CAD build for the part. Positions are in the model's coordinates, mm. Face numbers are marked on the shaded views. A direction names the side the tool comes from. Coordinates: 2 decimals unless noted, no trailing zeros. Write each loop counter-clockwise with the first axis right and the second up, starting at its lowest first coordinate (ties: lowest second). Pieces come first, ordered by that corner, then holes. Notation, with made-up numbers: (56.25, 20) - (65.25, 20) arc R7 ccw to (65.25, 26) - close; hole circle Ø4 at (-30.5, 80.25). An arc over 180 degrees is marked (long way). One line per question, with ' | ' between items. Start each with the question number.
1. Which spindle directions (+Z, -Z, +X, -X, +Y, -Y) get a long thin tool onto all of the face, cutting with end or side? Do the marked faces 1, 2 and 3. Say none if no direction does.
2. Probe line 1 (Z direction, x = -3.5, y = 4); line 2 (X direction, y = -22, z = -5); line 3 (X direction, y = -14, z = -11.5). List the from-to ranges inside material, lowest first.
3. Band-saw the part on A-A, the plane z = -6.35. Give the number of separate pieces and of enclosed holes in the cut face, then the cut area to 3 significant figures.
4. Flat gauge pins, fed straight in: P1, Ø6, axis at x = -19.5, z = -5, coming from the +Y side; P2, Ø4, axis at x = -22, y = -3.5, coming from the +Z side; P3, Ø0.8, axis at x = -31, z = -6.5, coming from the +Y side; P4, Ø1.4, axis at y = 5.5, z = -11, coming from the +X side. Where does each tip first touch, or does it go through?
5. Two-plate mould, pull along Z, no slides. Class the marked faces 4, 5, 6 and 7: +Z half, -Z half, draft (parallel to the pull), parting line (faces both ways), or undercut.
6. Band-saw the part on C-C, the plane x = 34.5. Write the cut outline in (y, z) (3 decimals), then the cut area to 3 significant figures.
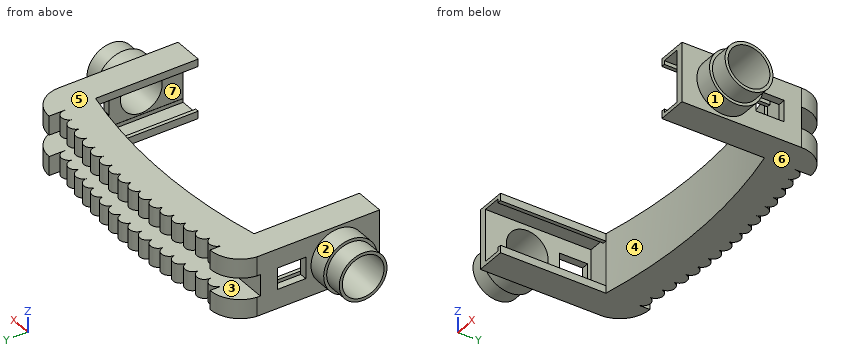
from build123d import *

# Parameters (mm, degrees)
BOSS_EXTRUDE1_DEPTH              = 12.7
SKETCH3_W                        = 4.569606656
SKETCH3_H                        = 12.610946307
CUT_EXTRUDE1_DEPTH               = 32.573497659
CUT_EXTRUDE1_DEPTH_BACK          = 32.704428158
SKETCH4_W                        = 4.569606656
SKETCH4_H                        = 6.0391821
CUT_EXTRUDE2_DEPTH               = 66.04
SKETCH5_R                        = 5.715
BOSS_EXTRUDE2_DEPTH              = 3.96875
SKETCH7_R                        = 5.09318723
BOSS_EXTRUDE3_DEPTH              = 3.96875
SKETCH9_R                        = 5.715
BOSS_EXTRUDE4_DEPTH              = 3.96875
SKETCH10_R                       = 5.08
BOSS_EXTRUDE5_DEPTH              = 3.96875
SKETCH8_R                        = 4.445
CUT_EXTRUDE4_DEPTH               = 80.152925816
CUT_EXTRUDE5_REACH               = 17.829
CUT_EXTRUDE5_OFFSET_FROM_SURFACE = 1.5875
SKETCH11_W                       = 9.525
SKETCH11_H                       = 24.345154454
SKETCH13_W                       = 9.525
SKETCH13_H                       = 22.482269966
CUT_EXTRUDE6_DEPTH               = 4.7625
CUT_EXTRUDE7_REACH               = 34.831
SKETCH14_W                       = 3.882511223
SKETCH14_H                       = 11.1125
SKETCH15_W                       = 3.945830838
SKETCH15_H                       = 11.1125
CUT_EXTRUDE8_DEPTH               = 22.48227


with BuildPart() as part:
    # Sketch1 → Boss-Extrude1 (new body)
    with BuildSketch(Plane.XY):
        with BuildLine():
            Line((25.223497659, -24.95432425), (31.573497659, -24.95432425))
            Line((31.573497659, -24.95432425), (31.573497659, 0.44567575))
            ThreePointArc((31.573497659, 0.44567575), (29.713625719, 4.935803811), (25.223497659, 6.79567575))
            Line((25.223497659, 6.79567575), (25.223497659, 3.36874218))
            ThreePointArc((25.223497659, 3.36874218), (25.194005143, 3.37526688), (25.164511033, 3.381784371))
            ThreePointArc((25.164511033, 3.381784371), (23.912297459, 5.232947026), (22.049913461, 3.997484421))
            ThreePointArc((22.049913461, 3.997484421), (20.787428344, 5.879791305), (18.929672437, 4.581449722))
            ThreePointArc((18.929672437, 4.581449722), (17.666399498, 6.401938478), (15.813867684, 5.186140916))
            ThreePointArc((15.813867684, 5.186140916), (14.370419451, 6.86745546), (12.652448322, 5.467835298))
            ThreePointArc((12.652448322, 5.467835298), (11.236710182, 7.228730664), (9.494148573, 5.790486593))
            ThreePointArc((9.494148573, 5.790486593), (8.033635968, 7.514426817), (6.328601682, 6.03188675))
            ThreePointArc((6.328601682, 6.03188675), (4.824278861, 7.717733664), (3.157897585, 6.191876393))
            ThreePointArc((3.157897585, 6.191876393), (1.610757722, 7.838516978), (-0.015870376, 6.270349895))
            ThreePointArc((-0.015870376, 6.270349895), (-1.604805836, 7.876697016), (-3.190606835, 6.267255447))
            ThreePointArc((-3.190606835, 6.267255447), (-4.820288856, 7.832248571), (-6.364215787, 6.182595092))
            ThreePointArc((-6.364215787, 6.182595092), (-8.033568431, 7.705200989), (-9.534601973, 6.016424724))
            ThreePointArc((-9.534601973, 6.016424724), (-11.24252311, 7.495638149), (-12.69967226, 5.76885405))
            ThreePointArc((-12.69967226, 5.76885405), (-14.466077033, 7.201365285), (-15.851850507, 5.398061056))
            ThreePointArc((-15.851850507, 5.398061056), (-17.628014087, 6.745603643), (-18.999984081, 4.988240156))
            ThreePointArc((-18.999984081, 4.988240156), (-20.801252814, 6.376658399), (-22.142035626, 4.539656571))
            ThreePointArc((-22.142035626, 4.539656571), (-23.987693231, 5.836740457), (-25.266933007, 3.978670437))
            ThreePointArc((-25.266933007, 3.978670437), (-25.282113604, 3.97569181), (-25.297293828, 3.972711283))
            Line((-25.297293828, 3.972711283), (-25.297293828, 6.794845101))
            ThreePointArc((-25.297293828, 6.794845101), (-29.574532825, 5.2306288), (-31.704428158, 1.205073937))
            Line((-31.704428158, 1.205073937), (-31.704428158, -24.95432425))
            Line((-31.704428158, -24.95432425), (-25.4, -24.95432425))
            Line((-25.4, -24.95432425), (-25.440666935, -2.463598833))
            ThreePointArc((-25.440666935, -2.463598833), (-0.075359426, 0.000928604), (25.223497659, -3.071619312))
            Line((25.223497659, -3.071619312), (25.223497659, -24.95432425))
        make_face()
    extrude(amount=-BOSS_EXTRUDE1_DEPTH)

    # Sketch3 → Cut-Extrude1 (cut, two sides)
    with BuildSketch(Plane(origin=(0, 0, 0), x_dir=(0, 0, -1), z_dir=(1, 0, 0))) as cut_extrude1_sk:
        with Locations((6.35, 6.751148903)):
            Rectangle(SKETCH3_W, SKETCH3_H)
    extrude(amount=CUT_EXTRUDE1_DEPTH, mode=Mode.SUBTRACT)
    extrude(cut_extrude1_sk.sketch, amount=-CUT_EXTRUDE1_DEPTH_BACK, mode=Mode.SUBTRACT)

    # Sketch4 → Cut-Extrude2 (cut)
    with BuildSketch(Plane(origin=(31.573497659, 0, 0), x_dir=(0, 0, -1), z_dir=(1, 0, 0))):
        with Locations((6.35, -6.205492883)):
            Rectangle(SKETCH4_W, SKETCH4_H)
    extrude(amount=-CUT_EXTRUDE2_DEPTH, mode=Mode.SUBTRACT)

    # Sketch5 → Boss-Extrude2 (add)
    with BuildSketch(Plane(origin=(31.573497659, 0, 0), x_dir=(0, 0, -1), z_dir=(1, 0, 0))):
        with Locations((6.35, -16.06432425)):
            Circle(SKETCH5_R)
    extrude(amount=BOSS_EXTRUDE2_DEPTH)

    # Sketch7 → Boss-Extrude3 (add)
    with BuildSketch(Plane(origin=(35.542247659, 0, 0), x_dir=(0, 0, -1), z_dir=(1, 0, 0))):
        with Locations((6.35, -16.06432425)):
            Circle(SKETCH7_R)
    extrude(amount=BOSS_EXTRUDE3_DEPTH)

    # Sketch9 → Boss-Extrude4 (add)
    with BuildSketch(Plane.ZY.offset(31.704428158)):
        with Locations((-6.35, -16.06432425)):
            Circle(SKETCH9_R)
    extrude(amount=BOSS_EXTRUDE4_DEPTH)

    # Sketch10 → Boss-Extrude5 (add)
    with BuildSketch(Plane.ZY.offset(35.673178158)):
        with Locations((-6.35, -16.06432425)):
            Circle(SKETCH10_R)
    extrude(amount=BOSS_EXTRUDE5_DEPTH)

    # Sketch8 → Cut-Extrude4 (cut, through all)
    with BuildSketch(Plane(origin=(39.510997659, 0, 0), x_dir=(0, 0, -1), z_dir=(1, 0, 0))):
        with Locations((6.35, -16.06432425)):
            Circle(SKETCH8_R)
    extrude(amount=-CUT_EXTRUDE4_DEPTH, mode=Mode.SUBTRACT)

    # Cut-Extrude5: up to this face of the body (flat: up to its plane, moved by the offset)
    cut_extrude5_end = Plane(part.part.faces().sort_by_distance((-31.704428158, -11.874625156, -0.290792729))[0]).offset(-CUT_EXTRUDE5_OFFSET_FROM_SURFACE)
    # Sketch11 → Cut-Extrude5 (cut, up to the picked face)
    with BuildSketch(Plane(origin=(-25.445038336, -0.046008819, 0), x_dir=(0, 0, -1), z_dir=(0.999998365, 0.001808162, 0)), mode=Mode.PRIVATE) as cut_extrude5_sk1:
        with Locations((6.35, -14.590171194)):
            Rectangle(SKETCH11_W, SKETCH11_H)
    cut_extrude5_tool1 = split(extrude(cut_extrude5_sk1.sketch, amount=-CUT_EXTRUDE5_REACH, mode=Mode.PRIVATE), bisect_by=cut_extrude5_end, keep=Keep.BOTH, mode=Mode.PRIVATE)
    add(cut_extrude5_tool1.solids().sort_by_distance((-25.418657, -14.636156, -6.35))[0], mode=Mode.SUBTRACT)

    # Sketch13 → Cut-Extrude6 (cut)
    with BuildSketch(Plane.ZY.offset(-25.223497659)):
        with Locations((-6.35, -13.713189267)):
            Rectangle(SKETCH13_W, SKETCH13_H)
    extrude(amount=-CUT_EXTRUDE6_DEPTH, mode=Mode.SUBTRACT)

    # Cut-Extrude7: up to this face of the body (flat: up to its plane)
    cut_extrude7_end = Plane(part.part.faces().sort_by_distance((-27.778797546, -2.467826558, -6.35))[0])
    # Sketch14 → Cut-Extrude7 (cut, up to the picked face)
    with BuildSketch(Plane.XZ.offset(24.95432425), mode=Mode.PRIVATE) as cut_extrude7_sk1:
        with Locations((-28.175672547, -6.35)):
            Rectangle(SKETCH14_W, SKETCH14_H)
    cut_extrude7_tool1 = split(extrude(cut_extrude7_sk1.sketch, amount=-CUT_EXTRUDE7_REACH, mode=Mode.PRIVATE), bisect_by=cut_extrude7_end, keep=Keep.BOTH, mode=Mode.PRIVATE)
    add(cut_extrude7_tool1.solids().sort_by_distance((-28.175673, -24.954324, -6.35))[0], mode=Mode.SUBTRACT)

    # Sketch15 → Cut-Extrude8 (cut)
    with BuildSketch(Plane.XZ.offset(24.95432425)):
        with Locations((27.990163078, -6.35)):
            Rectangle(SKETCH15_W, SKETCH15_H)
    extrude(amount=-CUT_EXTRUDE8_DEPTH, mode=Mode.SUBTRACT)


solid = part.part
Filled in:
1) face 1: +X | face 2: -X | face 3: +X, -X, +Y
2) line 1: z = -12.7 to -8.63, -4.07 to 0 | line 2: x = -31.7 to -30.12, 29.99 to 31.57 | line 3: x = -35.67 to -30.12, -26.23 to -25.42, 25.22 to 26.02, 29.96 to 35.54
3) separate pieces: 5 | enclosed holes: 0 | area: 160 mm²
4) P1: stops at y = 6.76 | P2: stops at z = 0 | P3: stops at y = 0.45 | P4: stops at x = 29.85
5) face 4: draft | face 5: +Z half | face 6: -Z half | face 7: undercut
6) outline: circle Ø11.43 at (-16.064, -6.35); hole circle Ø8.89 at (-16.064, -6.35) | area: 40.5 mm²
